Check sheet for the drawn part. Datum: minimum x, y, z corner. Units: mm. A direction names the side the tool comes from. Coordinates: 2 decimals unless noted, no trailing zeros. Write each loop counter-clockwise with the first axis right and the second up, starting at its lowest first coordinate (ties: lowest second). Pieces come first, ordered by that corner, then holes. Notation, with made-up numbers: (4.5, 44.25) -> (47.5, 44.25) arc R20 cw to (47.5, 64.25) -> close; hole circle Ø5 at (-5.75, 85.5). An arc over 180 degrees is marked (long way). Answer in a Markdown table with one row per item. Add a question column.
1. Cross-section at C-C on x = 12.7. Record the cut outline in (y, z), and give its area (3 significant figures).
2. Mould release check, pull along Z, two halves, no side actions. Record for the marked faces 3, 4, 5 and 6: pulls with the +Z half, pulls with the -Z half, needs draft (parallel to the pull), parting line crosses it, or undercut.
3. Cross-section at A-A on y = 46.99. Record the cut outline in (x, z).
4. Set-up check for the marked faces 1 and 2: record each of +Z, -Z, +X, -X, +Y, -Y from which the full face is reachable in a straight line by a thin tool's end or side.
5. Cross-section at D-D on y = 10.5. Record the cut outline in (x, z), and give its area (3 significant figures).
6. Scan lines: L1, parallel to Z at x = 1.2, y = 46.99; L2, parallel to X at y = 19, z = 17.75; L3, parallel to Y at x = 24.4, z = 3.81. Record each from-to range of solid material in increasing order. Write a range as from..to.
7. Cross-section at B-B on z = 3.81. Record the cut outline in (x, y), and give its area (3 significant figures).
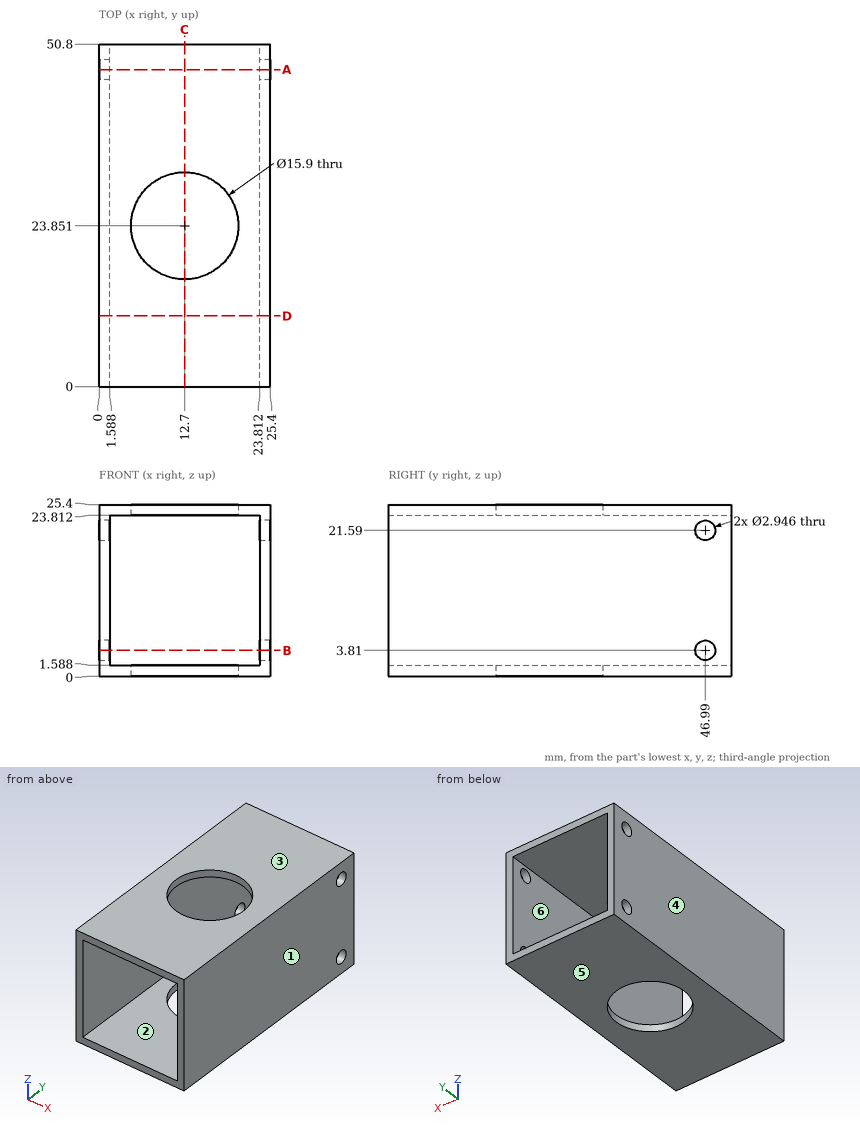
Results found:
| question | item | result |
|---|---|---|
| 1 | outline | (0, 0) -> (15.9, 0) -> (15.9, 1.59) -> (0, 1.59) -> close; (0, 23.81) -> (15.9, 23.81) -> (15.9, 25.4) -> (0, 25.4) -> close; (31.8, 0) -> (50.8, 0) -> (50.8, 1.59) -> (31.8, 1.59) -> close; (31.8, 23.81) -> (50.8, 23.81) -> (50.8, 25.4) -> (31.8, 25.4) -> close |
| 1 | area | 111 mm^2 |
| 2 | face 3 | pulls with the +Z half |
| 2 | face 4 | needs draft |
| 2 | face 5 | pulls with the -Z half |
| 2 | face 6 | undercut |
| 3 | outline | (0, 0) -> (25.4, 0) -> (25.4, 2.34) -> (23.81, 2.34) -> (23.81, 1.59) -> (1.59, 1.59) -> (1.59, 2.34) -> (0, 2.34) -> close; (0, 5.28) -> (1.59, 5.28) -> (1.59, 20.12) -> (0, 20.12) -> close; (0, 23.06) -> (1.59, 23.06) -> (1.59, 23.81) -> (23.81, 23.81) -> (23.81, 23.06) -> (25.4, 23.06) -> (25.4, 25.4) -> (0, 25.4) -> close; (23.81, 5.28) -> (25.4, 5.28) -> (25.4, 20.12) -> (23.81, 20.12) -> close |
| 4 | face 1 | +Z, -Z, +X, +Y, -Y |
| 4 | face 2 | +Y, -Y |
| 5 | outline | (0, 0) -> (25.4, 0) -> (25.4, 25.4) -> (0, 25.4) -> close; hole (1.59, 1.59) -> (23.81, 1.59) -> (23.81, 23.81) -> (1.59, 23.81) -> close |
| 5 | area | 151 mm^2 |
| 6 | L1 | z = 0..2.34, 5.28..20.12, 23.06..25.4 |
| 6 | L2 | x = 0..1.59, 23.81..25.4 |
| 6 | L3 | y = 0..45.52, 48.46..50.8 |
| 7 | outline | (0, 0) -> (1.59, 0) -> (1.59, 45.52) -> (0, 45.52) -> close; (0, 48.46) -> (1.59, 48.46) -> (1.59, 50.8) -> (0, 50.8) -> close; (23.81, 0) -> (25.4, 0) -> (25.4, 45.52) -> (23.81, 45.52) -> close; (23.81, 48.46) -> (25.4, 48.46) -> (25.4, 50.8) -> (23.81, 50.8) -> close |
| 7 | area | 152 mm^2 |
